from build123d import *

# Parameters (mm, degrees)
CIRPATTERN1_COUNT = 3


with BuildPart() as part:
    # Sketch2 → Revolve1 (revolve)
    with BuildSketch(Plane(origin=(0, 0, 0), x_dir=(0, 0, -1), z_dir=(1, 0, 0)), mode=Mode.PRIVATE) as revolve1_sk:
        with BuildLine():
            Line((9.0043, 3.4925), (9.0043, 6.87397239))
            ThreePointArc((9.0043, 6.87397239), (9.047344167, 7.018310977), (9.162415, 7.115497042))
            ThreePointArc((9.162415, 7.115497042), (10.0584, 7.3025), (10.954385, 7.115497042))
            ThreePointArc((10.954385, 7.115497042), (11.069455833, 7.018310977), (11.1125, 6.87397239))
            Line((11.1125, 6.87397239), (11.1125, 0))
            Line((11.1125, 0), (-11.1125, 0))
            Line((-11.1125, 0), (-11.1125, 1.905))
            Line((-11.1125, 1.905), (-9.8425, 3.175))
            Line((-9.8425, 3.175), (8.6868, 3.175))
            ThreePointArc((8.6868, 3.175), (8.911306403, 3.267993597), (9.0043, 3.4925))
        make_face()
    revolve(revolve1_sk.sketch.rotate(Axis((0, 0, -11.1125), (0, 0, 1)), 90), axis=Axis((0, 0, -11.1125), (0, 0, 1)))

    # Sketch4 → Revolve2 (revolve)
    with BuildSketch(Plane(origin=(0, 0, 0), x_dir=(0, 0, -1), z_dir=(1, 0, 0))):
        with BuildLine():
            Line((9.0043, -6.511925), (9.0043, -5.178425))
            Line((9.0043, -5.178425), (7.9375, -5.178425))
            ThreePointArc((7.9375, -5.178425), (8.237016729, -6.032281617), (9.0043, -6.511925))
        make_face()
    revolve2 = revolve(axis=Axis((0, -5.178425, -9.0043), (0, 0, 1)))

    # CirPattern1: Revolve2 ×3 about axis
    cirpattern1_axis = Axis((0, 0, 0), (0, 0, 1))
    for i in range(1, CIRPATTERN1_COUNT):
        add(revolve2.rotate(cirpattern1_axis, i * 360 / CIRPATTERN1_COUNT))


solid = part.part
Verification items for the finished model (mm, model axes). A direction names the side the tool comes from. Coordinates: 2 decimals unless noted, no trailing zeros. Write each loop counter-clockwise with the first axis right and the second up, starting at its lowest first coordinate (ties: lowest second). Pieces come first, ordered by that corner, then holes. Notation, with made-up numbers: (80, 3) -> (102, 3) arc R22 ccw to (102, 33) -> close; hole circle Ø7 at (-5, 39.5). An arc over 180 degrees is marked (long way). One line per item, written item: value. Start each with the question number.
Q1. Go/stop test with flat-tipped pins: P1, Ø8, axis at x = -6, z = 3, coming from the -Y side; P2, Ø7, axis at x = 1.5, y = -1.5, coming from the +Z side; P3, Ø5, axis at y = -4, z = -5, coming from the +X side; P4, Ø4, axis at y = -0.5, z = -5, coming from the -X side (3 decimals). Record where each tip stops, or that it passes through.
Q2. Access from +Z, -Z, +X, -X, +Y, -Y to the whole of each face (thin tool, end or side, straight path). Record for faces 1 (the flat face through (0, 0, -11.112)), 2 (the flat face through (3, 3, -9.004)).
Q3. Cross-section at C-C on z = -7.5. Enter the section's corners in (x, y) (3 decimals).
Q4. Thickness scan on L1, parallel to Z at x = -3.75, y = -3; L2, parallel to X at y = -1.5, z = -6.5; L3, parallel to Z at x = 0, y = -4.75. Record the ranges inside material, lowest first. Write a range as from..to.
Checked values:
1. P1: stops at y = -2.47
1. P2: stops at z = 11.11
1. P3: stops at x = 2.8
1. P4: stops at x = -3.175
2. face 1: -Z, +X, -X, +Y, -Y
2. face 2: +Z
3. outline: circle Ø6.35 at (0, 0)
4. L1: z = -11.11..-9
4. L2: x = -2.8..2.8
4. L3: z = -11.11..-8.01
